Part model, mm, in its own coordinate system. Round coordinates to 2 decimals unless told otherwise and drop trailing zeros. Order: outer loops, then holes, each group sorted by start corner. A loop starts at its lowest first (then second) coordinate and runs counter-clockwise, first axis right, second up. Notation, with made-up numbers: (-10, -34) -> (18, -34) arc R27 cw to (18, -3) -> close; hole circle Ø4 at (82.25, 18). An arc over 180 degrees is marked (long way). Use CSV: the item, a comma, the result in double quotes.
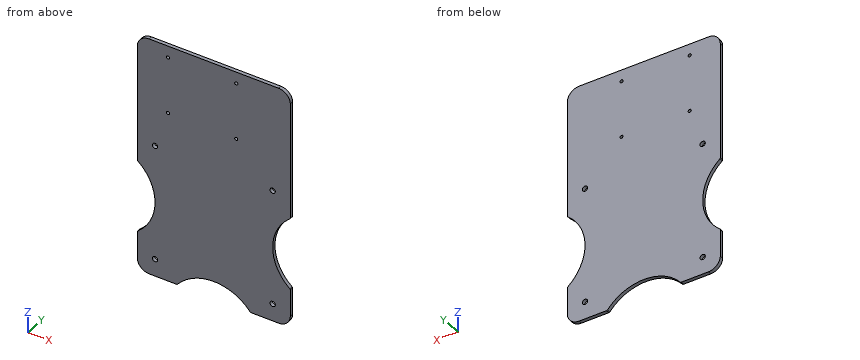
```python
from build123d import *

# Parameters (mm, degrees)
F0_R     = 2.25
F0_R_2   = 1.35
F0_R_3   = 1.3110502125
F1_DEPTH = 3
F2_R     = 1


with BuildPart() as f1:
    # F0 (on Front) → F1 (new body)
    with BuildSketch(Plane.XZ):
        with BuildLine():
            ThreePointArc((0, 10), (2.9289321881, 2.9289321881), (10, 0))
            Line((10, 0), (33.775010008, 0))
            ThreePointArc((33.775010008, 0), (65, 15), (96.224989992, 0))
            Line((96.224989992, 0), (120, 0))
            ThreePointArc((120, 0), (127.0710678119, 2.9289321881), (130, 10))
            Line((130, 10), (130, 33.775010008))
            ThreePointArc((130, 33.775010008), (115, 65), (130, 96.224989992))
            Line((130, 96.224989992), (130, 197.5))
            ThreePointArc((130, 197.5), (127.0710678119, 204.5710678119), (120, 207.5))
            Line((120, 207.5), (10, 207.5))
            ThreePointArc((10, 207.5), (2.9289321881, 204.5710678119), (0, 197.5))
            Line((0, 197.5), (0, 96.224989992))
            ThreePointArc((0, 96.224989992), (15, 65), (0, 33.775010008))
            Line((0, 33.775010008), (0, 10))
        make_face()
        with Locations((15, 15)):
            Circle(F0_R, mode=Mode.SUBTRACT)
        with Locations((115, 15)):
            Circle(F0_R, mode=Mode.SUBTRACT)
        with Locations((15, 115)):
            Circle(F0_R, mode=Mode.SUBTRACT)
        with Locations((26, 148.5)):
            Circle(F0_R_2, mode=Mode.SUBTRACT)
        with Locations((26, 197.5)):
            Circle(F0_R_2, mode=Mode.SUBTRACT)
        with Locations((84, 148.5)):
            Circle(F0_R_3, mode=Mode.SUBTRACT)
        with Locations((115, 115)):
            Circle(F0_R, mode=Mode.SUBTRACT)
        with Locations((84, 197.5)):
            Circle(F0_R_2, mode=Mode.SUBTRACT)
    extrude(amount=F1_DEPTH)

    # F2
    f2_edges = [f1.edges().sort_by_distance(p)[0] for p in [
        (0, -1.5, 33.77501),
        (130, -1.5, 96.22499),
        (33.77501, -1.5, 0),
        (96.22499, -1.5, 0),
        (130, -1.5, 33.77501),
        (0, -1.5, 96.22499),
    ]]
    fillet(f2_edges, radius=F2_R)


solid = f1.part
```
(1) Probe probe 1 along X at (y, z) = (-2.3, 148.5); probe 2 along Z at (x, y) = (26, -1.6); probe 3 along Z at (x, y) = (47.5, -2.5). List the from-to ranges inside material, lowest first. Write a range as [from, to].
Reply:
probe 1,"[0, 24.65], [27.35, 82.69], [85.31, 130]"
probe 2,"[0, 147.15], [149.85, 196.15], [198.85, 207.5]"
probe 3,"[10.97, 207.5]"
(2) Cut at B-B, the plane z = 41. Give the cut face in (x, y), then the cut area to 3 significant figures.
Reply:
outline,"(7, -3) -> (123, -3) -> (123, 0) -> (7, 0) -> close"
area,"348 mm2"
(3) Cut at A-A, the plane y = -1.15. State how many separate pieces and enclosed holes the cut face has, then the cut area to 3 significant figures.
Reply:
separate pieces,"1"
enclosed holes,"8"
area,"24,800 mm2"
(4) Cut at C-C, the plane x = 89. Give the cut face in (y, z).
Reply:
outline,"(-3, 7) -> (0, 7) -> (0, 207.5) -> (-3, 207.5) -> close"
